Design review of the part built by this model. Coordinates are the model's own, in mm. Round coordinates to 2 decimals unless told otherwise and drop trailing zeros. Write each loop counter-clockwise with the first axis right and the second up, starting at its lowest first coordinate (ties: lowest second). Pieces come first, ordered by that corner, then holes. Notation, with made-up numbers: (72, 18.25) -> (116, 18.25) arc R24 ccw to (116, 49.25) -> close; hole circle Ø3 at (5.5, -12.75). An arc over 180 degrees is marked (long way). One line per question, with ' | ' between items. Start each with the question number.
1) Consider section D-D (x = 157). Give the boundary of the cut face in (y, z), then the cut area to 3 significant figures.
2) Consider section A-A (x = 50). Give the boundary of the cut face in (y, z).
3) Consider section B-B (y = 0). Give the boundary of the cut face in (x, z), then the cut area to 3 significant figures.
4) Consider section C-C (z = 3.5). Give the boundary of the cut face in (x, y), then the cut area to 3 significant figures.
5) For probe 1 along Y at (x, z) = (50, 4.5); probe 2 along Y at (x, z) = (155, 2.5); probe 3 along X at (y, z) = (10.5, 3), list the stretches that pass through material, from the lowest coordinate up.
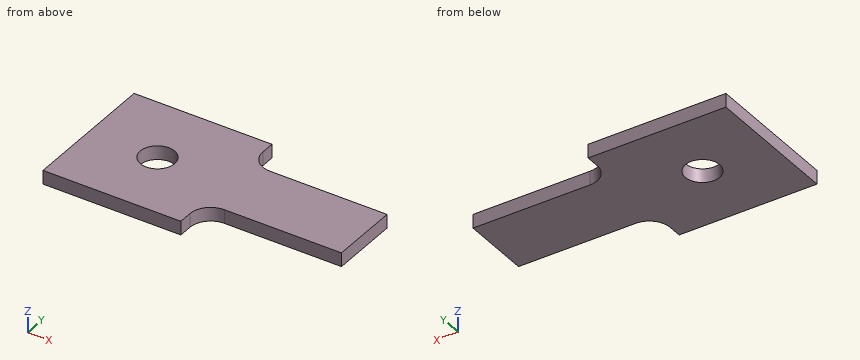
```python
from build123d import *

# Parameters (mm, degrees)
BOSS_EXTRUDE1_DEPTH = 10
SKETCH2_R           = 12.5
CUT_EXTRUDE1_DEPTH  = 11


with BuildPart() as part:
    # Sketch1 → Boss-Extrude1 (new body)
    with BuildSketch(Plane.XY):
        with BuildLine():
            Line((200, -25), (200, 25))
            Line((200, 25), (115, 25))
            ThreePointArc((115, 25), (104.393398282, 29.393398282), (100, 40))
            Line((100, 40), (100, 50))
            Line((100, 50), (0, 50))
            Line((0, 50), (0, -50))
            Line((0, -50), (100, -50))
            Line((100, -50), (100, -40))
            ThreePointArc((100, -40), (104.393398282, -29.393398282), (115, -25))
            Line((115, -25), (200, -25))
        make_face()
    extrude(amount=BOSS_EXTRUDE1_DEPTH)

    # Sketch2 → Cut-Extrude1 (cut, through all)
    with BuildSketch(Plane.XY.offset(10)):
        with Locations((50, 0)):
            Circle(SKETCH2_R)
    extrude(amount=-CUT_EXTRUDE1_DEPTH, mode=Mode.SUBTRACT)


solid = part.part
```
From the geometry:
1) outline: (-25, 0) -> (25, 0) -> (25, 10) -> (-25, 10) -> close | area: 500 mm2
2) outline: (-50, 0) -> (-12.5, 0) -> (-12.5, 10) -> (-50, 10) -> close; (12.5, 0) -> (50, 0) -> (50, 10) -> (12.5, 10) -> close
3) outline: (0, 0) -> (37.5, 0) -> (37.5, 10) -> (0, 10) -> close; (62.5, 0) -> (200, 0) -> (200, 10) -> (62.5, 10) -> close | area: 1,750 mm2
4) outline: (0, -50) -> (100, -50) -> (100, -40) arc R15 cw to (115, -25) -> (200, -25) -> (200, 25) -> (115, 25) arc R15 cw to (100, 40) -> (100, 50) -> (0, 50) -> close; hole circle Ø25 at (50, 0) | area: 14,600 mm2
5) probe 1: y = -50 to -12.5, 12.5 to 50 | probe 2: y = -25 to 25 | probe 3: x = 0 to 43.22, 56.78 to 200
